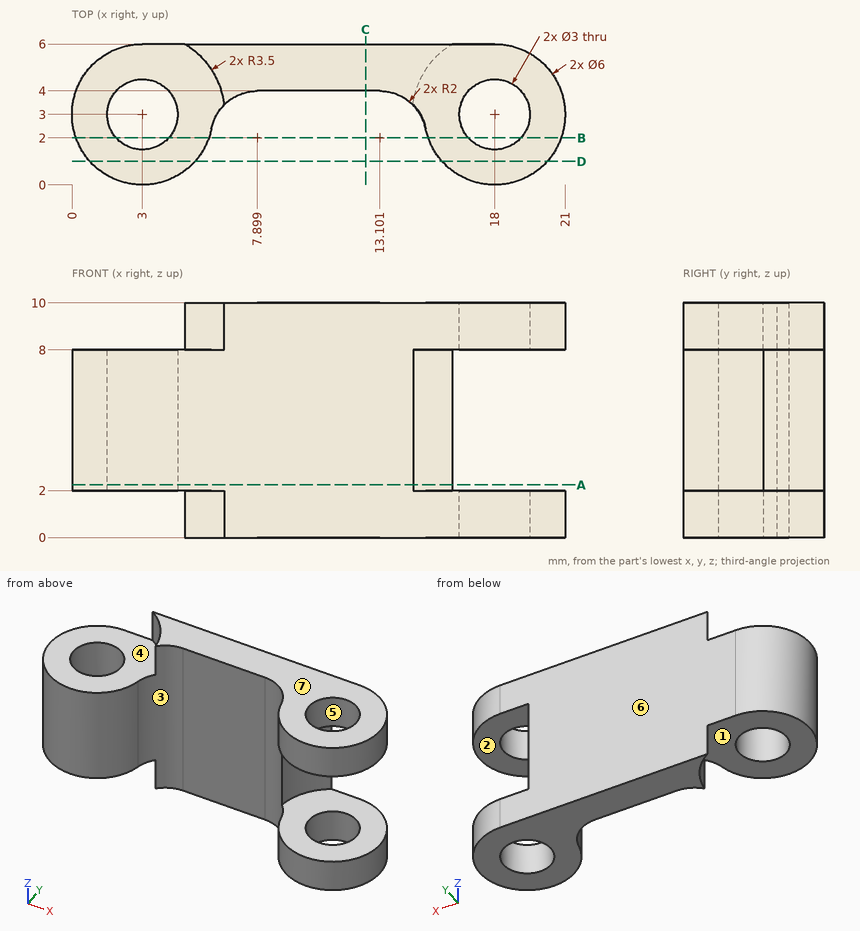
Source: three-view drawing plus pictorial views. Frame: mm from the lowest corner of the part. A direction names the side the tool comes from. Coordinates: 2 decimals unless noted, no trailing zeros. Order: outer loops, then holes, each group sorted by start corner. A loop starts at its lowest first (then second) coordinate and runs counter-clockwise, first axis right, second up. Notation, with made-up numbers: M 67,10.5 L 123,10.5 A14 cw 123,24.5 Z; hole C 48,67.25 d6. An arc over 180 degrees is marked long. One line per question, with ' | ' between items. Start each with the question number.
Item 1: Cut plane A-A, the plane z = 2.25. Return the cut outline in (x, y), then the cut area to 3 significant figures.
Item 2: Cut plane B-B, the plane y = 2. Return the cut outline in (x, z), then the cut area to 3 significant figures.
Item 3: Cut plane D-D, the plane y = 1. Return the cut outline in (x, z).
Item 4: Ray query, probe 1 along Y at (x, z) = (3, 5.5); probe 2 along Z at (x, y) = (19.5, 5.5); probe 3 along Y at (x, z) = (12.75, 4.25). Return the intervals inside material, ascending. Write a range as [from, to].
Item 5: Cut plane C-C, the plane x = 12.5. Return the cut outline in (y, z).
Item 6: Set-up query: the marked faces 1, 2, 3 and 4. Return all of +Z, -Z, +X, -X, +Y, -Y with unobstructed straight access to the full face (end or side cutting, diameter ignored); none if empty.
Item 7: Pin query (flat end, axial travel): pin 1 Ø1.5 at (x, y) = (16, 2.5) entering from -Z; pin 2 Ø1.8 at (x, y) = (4, 3.5) entering from +Z; pin 3 Ø1 at (x, y) = (2.5, 3) entering from +Z; pin 4 Ø4 at (x, z) = (10, 4.5) entering from -Y. Return the tip coordinate at first contact, or that it passes through.
Item 8: Draft query along Y for the marked faces 5, 6 and 7. Return one class per face: released by +Y, released by -Y, zero draft, split by the parting line, or undercut.
A:
1) outline: M 3,6 A3 ccw long 5.94,2.4 A2 cw 7.9,4 L 13.1,4 A2 cw 14.52,3.41 A3.5 cw 16.2,6 Z; hole C 3,3 d3 | area: 42.6 mm2
2) outline: M 0.17,2 L 1.88,2 L 1.88,8 L 0.17,8 Z; M 4.12,2 L 5.83,2 L 5.83,8 L 4.12,8 Z; M 15.17,0 L 16.88,0 L 16.88,2 L 15.17,2 Z; M 15.17,8 L 16.88,8 L 16.88,10 L 15.17,10 Z; M 19.12,0 L 20.83,0 L 20.83,2 L 19.12,2 Z; M 19.12,8 L 20.83,8 L 20.83,10 L 19.12,10 Z | area: 34.2 mm2
3) outline: M 0.76,2 L 5.24,2 L 5.24,8 L 0.76,8 Z; M 15.76,0 L 20.24,0 L 20.24,2 L 15.76,2 Z; M 15.76,8 L 20.24,8 L 20.24,10 L 15.76,10 Z
4) probe 1: y = [0, 1.5], [4.5, 6] | probe 2: z = [0, 2], [8, 10] | probe 3: y = [4, 6]
5) outline: M 4,0 L 6,0 L 6,10 L 4,10 Z
6) face 1: -Z, -X, -Y | face 2: +X, -Y | face 3: +Z, -Z, -Y | face 4: +Z, -X, -Y
7) pin 1: stops at z = 0 | pin 2: stops at z = 8 | pin 3: passes through | pin 4: stops at y = 4
8) face 5: undercut | face 6: released by +Y | face 7: zero draft
